Autodesk Inventor part; units mm, degrees
ref_plane "YZ Plane" through (0, 0, 0) normal (1, 0, 0) x (0, 1, 0)
ref_plane "XZ Plane" through (0, 0, 0) normal (0, 1, 0) x (-1, 0, 0)
ref_plane "XY Plane" through (0, 0, 0) normal (0, 0, 1) x (1, 0, 0)
sketch "Sketch1" plane through (0, 0, 0) normal (0, 1, 0) x (-1, 0, 0)
  line L0 (-29.4449, -51) -> (-58.8897, 0)
  line L1 (-58.8897, 0) -> (-29.4449, 51)
  line L2 (-29.4449, 51) -> (29.4449, 51)
  line L3 (29.4449, 51) -> (58.8897, 0)
  line L4 (58.8897, 0) -> (29.4449, -51)
  line L5 (29.4449, -51) -> (-29.4449, -51)
  line L6 (-31.2924, -54.2) -> (-62.5848, 0)
  line L7 (-62.5848, 0) -> (-31.2924, 54.2)
  line L8 (-31.2924, 54.2) -> (31.2924, 54.2)
  line L9 (31.2924, 54.2) -> (62.5848, 0)
  line L10 (62.5848, 0) -> (31.2924, -54.2)
  line L11 (31.2924, -54.2) -> (-31.2924, -54.2)
  line L12 (-30.3109, -52.5) -> (-60.6218, 0)
  line L13 (-60.6218, 0) -> (-30.3109, 52.5)
  line L14 (-30.3109, 52.5) -> (30.3109, 52.5)
  line L15 (30.3109, 52.5) -> (60.6218, 0)
  line L16 (60.6218, 0) -> (30.3109, -52.5)
  line L17 (30.3109, -52.5) -> (-30.3109, -52.5)
  line L18 (-30.4264, -52.7) -> (-60.8527, 0)
  line L19 (-60.8527, 0) -> (-30.4264, 52.7)
  line L20 (-30.4264, 52.7) -> (30.4264, 52.7)
  line L21 (30.4264, 52.7) -> (60.8527, 0)
  line L22 (60.8527, 0) -> (30.4264, -52.7)
  line L23 (30.4264, -52.7) -> (-30.4264, -52.7)
  line L24 (0, -51) -> (0, -52.5) construction
  line L25 (0, -52.7) -> (0, -54.2) construction
  line L26 (28.8675, 50) -> (39.5485, 31.5)
  line L27 (39.5485, 31.5) -> (14.7224, 31.5)
  line L28 (14.7224, 31.5) -> (4.0415, 50)
  line L29 (4.0415, 50) -> (28.8675, 50)
  line L30 (-29.1562, 50.5) -> (29.1562, 50.5) construction
  line L31 (29.1562, 50.5) -> (58.3124, 0) construction
  line L32 (58.3124, 0) -> (29.1562, -50.5) construction
  line L33 (29.1562, -50.5) -> (-29.1562, -50.5) construction
  line L34 (-29.1562, -50.5) -> (-58.3124, 0) construction
  line L35 (-58.3124, 0) -> (-29.1562, 50.5) construction
  line L36 (40.2124, 30.35) -> (14.0007, 30.35) construction
  line L37 (14.0007, 30.35) -> (2.6558, 50) construction
  point P0 (0, 0)
  point P1 (0, 0)
  point P2 (0, 0)
  dimension "d0" = 102
  dimension "d1" = 3.2
  dimension "d2" = 0.2
  dimension "d3" = 1
  dimension "d4" = 1
  dimension "d5" = 101
  dimension "d6" = 19
  dimension "d7" = 21.5
  dimension "Outside" = 108.4
  dimension "d17" = 20.15
  dimension "d18" = 23.2
  dimension "d19" = 1.15
  dimension "d20" = 1.2
extrude "Extrusion1" add sketch "Sketch1" along normal blind 1 contours L0 L1 L2 L3 L4 L5 | L6 L7 L8 L9 L10 L11 | L12 L13 L14 L15 L16 L17 | L18 L19 L20 L21 L22 L23
extrude "Extrusion2" add sketch "Sketch1" against normal blind 2.8 contours L6 L7 L8 L9 L10 L11
fillet "Fillet1" radius 2 2 edges at (-28.8675, 0.5, 50) (-14.7224, 0.5, 31.5)
fillet "Fillet1" radius 1 2 edges at (-39.5485, 0.5, 31.5) (-4.0415, 0.5, 50)
fillet "Fillet1" radius 2 6 edges at (-31.2924, -0.9, 54.2) (31.2924, -0.9, 54.2) (62.5848, -0.9, 0) (31.2924, -0.9, -54.2) (-31.2924, -0.9, -54.2) (-62.5848, -0.9, 0)
chamfer "Chamfer1" distance 1 angle 45 12 edges at (-46.9386, 1, -27.1) (-62.2754, 1, 0) (-46.9386, 1, 27.1) (-31.1377, 1, 53.9321) (0, 1, 54.2) (31.1377, 1, 53.9321) (46.9386, 1, 27.1) (62.2754, 1, 0) (46.9386, 1, -27.1) (31.1377, 1, -53.9321) (0, 1, -54.2) (-31.1377, 1, -53.9321)
equation "\"d0\" = Inside"
equation "\"d4\" = d3"
equation "\"d5\" = FlatDiameter"
equation "\"d17\" = CouncilHomeHeight"
equation "\"d18\" = CouncilHomeWidth"
equation "\"d8\" = FaceThickness"
equation "\"d10\" = LidDepth - Clearance"
equation "\"Clearance\" = 0.2"
equation "\"LidDepth\" = 3"
equation "\"FaceThickness\" = 1"
properties part number "Factions_Lid" material "ABS Plastic"
The model under review builds one solid part; all positions refer to its coordinate system, in mm. A direction names the side the tool comes from. Round coordinates to 2 decimals unless told otherwise and drop trailing zeros. Loops run counter-clockwise (first coordinate to the right, second up) from the corner with the lowest first, then second, coordinate; pieces in that order, holes last. Notation, with made-up numbers: (50, 80) -> (66, 80) arc R17 ccw to (66, 105) -> close; hole circle Ø4 at (65.25, 68). An arc over 180 degrees is marked (long way). One line per question, with ' | ' between items. Start each with the question number.
Item 1: Machinability: for faces 1 (the face through (-45.427, -1.38, 26.719)), 2 (the face through (-34, 0.49, 41.11)), 3 (the face through (46.728, -1.38, -27.465)), which of the approach directions +Z, -Z, +X, -X, +Y, -Y give a long, thin tool a straight path to every point of the face, cutting with its end or side? Answer none if there is none.
Item 2: Add section A-A, the plane y = -1.85. Write out the cut boundary in (x, z).
Item 3: Add section C-C, the plane z = 43. Write out the cut boundary in (x, y).
Item 4: Add section B-B, the plane x = -18. Write out the cut boundary in (y, z), then the cut area to 3 significant figures.
Item 5: For pin 1 (1 mm diameter, centred on y = 0.5, z = -43.5, fed in from +X); pin 2 (1.5 mm diameter, centred on x = 16, z = 25.5, fed in from -Y); pin 3 (0.5 mm diameter, centred on x = -21.5, y = 0.5, fed in from +Z), all flat-tipped, find the tip position at first contact; note any pin that passes through.
Item 6: Wall thickness on line 1 along Z through (x, y) = (-24, -0.3); line 2 along Y through (x, z) = (42.5, -1.5); line 3 along Z through (x, y) = (50, -1.15): over which ranges is each line inside the solid? List them lowest first. Write a range as [from, to].
Item 7: Add section D-D, the plane x = 24. Write out the cut boundary in (y, z).
Return value:
1) face 1: -Y | face 2: +Y, -Y | face 3: -Z, +X, +Y, -Y
2) outline: (-62.01, -1) -> (-31.87, -53.2) arc R2 ccw to (-30.14, -54.2) -> (30.14, -54.2) arc R2 ccw to (31.87, -53.2) -> (62.01, -1) arc R2 ccw to (62.01, 1) -> (31.87, 53.2) arc R2 ccw to (30.14, 54.2) -> (-30.14, 54.2) arc R2 ccw to (-31.87, 53.2) -> (-62.01, 1) arc R2 ccw to start; hole (-60.85, 0) -> (-30.43, -52.7) -> (30.43, -52.7) -> (60.85, 0) -> (30.43, 52.7) -> (-30.43, 52.7) -> close
3) outline: (-37.76, -2.8) -> (-36.03, -2.8) -> (-36.03, 0) -> (-32.91, 0) -> (-32.91, 1) -> (-36.6, 1) -> (-37.76, 0) -> close; (-8.08, 0) -> (36.03, 0) -> (36.03, -2.8) -> (37.76, -2.8) -> (37.76, 0) -> (36.6, 1) -> (-8.08, 1) -> close
4) outline: (-2.8, -54.2) -> (0, -54.2) -> (1, -53.2) -> (1, 31.5) -> (0, 31.5) -> (0, -52.7) -> (-2.8, -52.7) -> close; (-2.8, 52.7) -> (0, 52.7) -> (0, 50) -> (1, 50) -> (1, 53.2) -> (0, 54.2) -> (-2.8, 54.2) -> close | area: 97.3 mm2
5) pin 1: stops at x = 37.54 | pin 2: stops at y = 0 | pin 3: stops at z = 53.95
6) line 1: z = [-54.2, -52.7], [52.7, 54.2] | line 2: y = [0, 1] | line 3: z = [-21.8, -18.8], [18.8, 21.8]
7) outline: (-2.8, -54.2) -> (0, -54.2) -> (1, -53.2) -> (1, 53.2) -> (0, 54.2) -> (-2.8, 54.2) -> (-2.8, 52.7) -> (0, 52.7) -> (0, -52.7) -> (-2.8, -52.7) -> close
